```python
from build123d import *

# Parameters (mm, degrees)
SKETCH4_R           = 2.413
CUT_EXTRUDE1_DEPTH  = 1.27
BOSS_EXTRUDE1_START = 0.635
SKETCH3_R           = 2.413
BOSS_EXTRUDE1_DEPTH = 0.635


with BuildPart() as part:
    # Sketch2 → Revolve1 (revolve)
    with BuildSketch(Plane(origin=(0, 0, 0), x_dir=(0, 0, -1), z_dir=(1, 0, 0)), mode=Mode.PRIVATE) as revolve1_sk:
        Polygon((0, 3), (0, 6.35), (19.05, 6.35), (19.05, 3.96875), (9.525, 3.96875), (9.525, 3), align=None)
    revolve(revolve1_sk.sketch.rotate(Axis((0, 0, 0), (0, 0, -1)), 90), axis=Axis((0, 0, 0), (0, 0, -1)))

    # Sketch4 → Cut-Extrude1 (cut)
    with BuildSketch(Plane(origin=(0, 6.35, 0), x_dir=(1, 0, 0), z_dir=(0, 1, 0))):
        with Locations(Location((0, 3.81, 0), (0, 0, 270))):
            Circle(SKETCH4_R)
    cut_extrude1 = extrude(amount=-CUT_EXTRUDE1_DEPTH, mode=Mode.SUBTRACT)

    # Sketch3 → Boss-Extrude1 (add)
    with BuildSketch(Plane(origin=(0, 5.08, 0), x_dir=(1, 0, 0), z_dir=(0, 1, 0)).offset(BOSS_EXTRUDE1_START)):
        with Locations(Location((0, 3.81, 0), (0, 0, 270))):
            Circle(SKETCH3_R)
        Polygon((1.374815329, 3.81), (0.687407664, 5.000625), (-0.687407664, 5.000625), (-1.374815329, 3.81), (-0.687407664, 2.619375), (0.687407664, 2.619375), align=None, mode=Mode.SUBTRACT)
    boss_extrude1 = extrude(amount=-BOSS_EXTRUDE1_DEPTH)

    # Mirror1: Cut-Extrude1, Boss-Extrude1 across plane
    add(cut_extrude1.mirror(Plane.XY.offset(-9.525)), mode=Mode.SUBTRACT)
    add(boss_extrude1.mirror(Plane.XY.offset(-9.525)))


solid = part.part
```
CAD build for the part. Positions are in the model's coordinates, mm. A direction names the side the tool comes from. Give positions to 0.01 mm unless a question says otherwise; leave off trailing zeros. Write each loop counter-clockwise with the first axis right and the second up, starting at its lowest first coordinate (ties: lowest second). Pieces come first, ordered by that corner, then holes. Notation, with made-up numbers: M 67,-3.5 L 100,-3.5 A23 ccw 100,21.5 Z; hole C -10,29 d2. An arc over 180 degrees is marked long. Return JSON: item names as keys, results as strings. Group by question number.
(1) Band-saw the part on C-C (z = -9.75). Give the cut face in (x, y).
(2) Band-saw the part on A-A (y = 0). Give the cut face in (x, z) (3 decimals), and give its area (3 significant figures).
(3) Drill centre lines: L1, parallel to Z at x = 0, y = 5.95; L2, parallel to Y at x = 0, z = -12; L3, parallel to Y at x = 0, z = -16.5 (3 decimals). Where is each one in solid material? Low to high. Write a range as [from, to].
(4) Band-saw the part on D-D (x = -2). Give the cut face in (y, z) (3 decimals).
(5) Flat gauge pins, fed straight in: pin 1 Ø2 at (y, z) = (-1.5, -8.5) entering from +X; pin 2 Ø7 at (x, y) = (0, 0) entering from -Z (3 decimals); pin 3 Ø5 at (x, z) = (-5, -3.5) entering from +Y. Where does each tip first touch, or does it go through?
(6) Band-saw the part on B-B (x = 0). Give the cut face in (y, z) (3 decimals), and give its area (3 significant figures).
(7) 3-axis set-ups, long thin cutter, end or side, ignore diameter. For faces 4 (the face through (1, -3, -9.525)), 5 (the face through (-0.8, -6.3, -9.7)), 6 (the face through (-1, 5.715, -2.8)): which of +Z, -Z, +X, -X, +Y, -Y reach the whole face in a straight line?
(8) Mould opens along Z. For faces 1 (the face through (3, -3, -19.05)), 2 (the face through (0, 5.08, -15)), 3 (the face through (-3, 1, 0)) say: pulls with the +Z half, pulls with the -Z half, needs draft (parallel to the pull), parting line crosses it, or undercut.
Entries:
{
 "1": {"outline": "C 0,0 d12.7; hole C 0,0 d7.94"},
 "2": {"outline": "M -6.35,-19.05 L -3.969,-19.05 L -3.969,-9.525 L -3,-9.525 L -3,0 L -6.35,0 Z; M 3,-9.525 L 3.969,-9.525 L 3.969,-19.05 L 6.35,-19.05 L 6.35,0 L 3,0 Z", "area": "109 mm^2"},
 "3": {"L1": "z = [-19.05, -17.65], [-12.83, -6.22], [-1.4, 0]", "L2": "y = [-6.35, -3.97], [3.97, 6.35]", "L3": "y = [-6.35, -3.969], [3.969, 5.715]"},
 "4": {"outline": "M -6.027,-19.05 L -3.428,-19.05 L -3.428,-9.525 L -2.236,-9.525 L -2.236,0 L -6.027,0 Z; M 2.236,-9.525 L 3.428,-9.525 L 3.428,-19.05 L 6.027,-19.05 L 6.027,-16.59 L 5.715,-16.59 L 5.715,-13.89 L 6.027,-13.89 L 6.027,-5.16 L 5.715,-5.16 L 5.715,-2.46 L 6.027,-2.46 L 6.027,0 L 2.236,0 Z"},
 "5": {"pin 1": "stops at x = 6.33", "pin 2": "stops at z = -9.525", "pin 3": "stops at y = 5.84"},
 "6": {"outline": "M -6.35,-19.05 L -3.969,-19.05 L -3.969,-9.525 L -3,-9.525 L -3,0 L -6.35,0 Z; M 3,-9.525 L 3.969,-9.525 L 3.969,-19.05 L 6.35,-19.05 L 6.35,-17.653 L 5.715,-17.653 L 5.715,-16.431 L 5.08,-16.431 L 5.08,-14.049 L 5.715,-14.049 L 5.715,-12.827 L 6.35,-12.827 L 6.35,-6.223 L 5.715,-6.223 L 5.715,-5.001 L 5.08,-5.001 L 5.08,-2.619 L 5.715,-2.619 L 5.715,-1.397 L 6.35,-1.397 L 6.35,0 L 3,0 Z", "area": "100 mm^2"},
 "7": {"face 4": "-Z", "face 5": "+Z, -Z", "face 6": "+Y"},
 "8": {"face 1": "pulls with the -Z half", "face 2": "undercut", "face 3": "pulls with the +Z half"}
}
